Design review of the part built by this model. Coordinates are the model's own, in mm. Face numbers are marked on the shaded views. A direction names the side the tool comes from. Round coordinates to 2 decimals unless told otherwise and drop trailing zeros. Order: outer loops, then holes, each group sorted by start corner. A loop starts at its lowest first (then second) coordinate and runs counter-clockwise, first axis right, second up. Notation, with made-up numbers: M 64,5 L 75,5 A19 cw 75,26 Z; hole C -6.5,-40 d10. An arc over 180 degrees is marked long. Use a Markdown table: item, result. Add a question column.
(1) The part is to be moulded in two halves that separate along Y. For the marked faces 1, 2, 3 and 4, say which applies: released by +Y, released by -Y, zero draft, split by the parting line, or undercut.
(2) Take a section at C-C (z = 6.5). Write out the cut boundary in (x, y).
(3) Take a section at A-A (y = -29). Write out the cut boundary in (x, z), then the cut area to 3 significant figures.
(4) Machinability: for the marked faces 5, 6 and 7, which of the approach directions +Z, -Z, +X, -X, +Y, -Y give a long, thin tool a straight path to every point of the face, cutting with its end or side? Answer none if there is none.
(5) For pin 1 (4 mm diameter, centred on x = 37.5, z = 5.5, fed in from -Y); pin 2 (2.5 mm diameter, centred on x = -41, z = 6, fed in from -Y); pin 3 (1 mm diameter, centred on y = -3, z = 5.5, fed in from -X); pin 4 (4 mm diameter, centred on x = -30, y = -29.5, fed in from +Z), all flat-tipped, find the tip position at first contact; note any pin that passes through.
(6) Take a section at D-D (x = -36). Write out the cut boundary in (y, z), then the cut area to 3 significant figures.
(7) Take a section at B-B (y = -16). Write out the cut boundary in (x, z).
(8) To check wall thickness, follow probe 1 along X at (y, z) = (-28, 6); probe 2 along Y at (x, z) = (0.5, 6); probe 3 along X at (y, z) = (-10, 1.75). State the ranges of each line that lie inside material, in increasing order. Write a range as from..to.
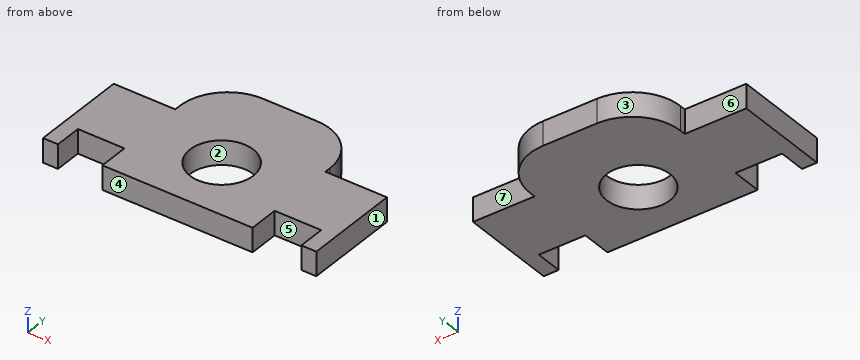
```python
from build123d import *

# Parameters (mm, degrees)
SKETCH2_W           = 70
SKETCH2_H           = 51
SKETCH2_R           = 10.55
BOSS_EXTRUDE1_DEPTH = 8
SKETCH3_W           = 10
SKETCH3_H           = 10
CUT_EXTRUDE1_DEPTH  = 53.436444721
SKETCH5_W           = 5.5
SKETCH5_H           = 8
BOSS_EXTRUDE2_DEPTH = 23
SKETCH5_3_W         = 5
SKETCH5_3_H         = 8
BOSS_EXTRUDE3_DEPTH = 32
SKETCH5_5_W         = 5
SKETCH5_5_H         = 8
BOSS_EXTRUDE4_DEPTH = 32
SKETCH5_6_W         = 5.5
SKETCH5_6_H         = 8
BOSS_EXTRUDE5_DEPTH = 23


with BuildPart() as part:
    # Sketch2 → Boss-Extrude1 (new body)
    with BuildSketch(Plane.XY):
        with Locations((1.074313409, -11.705169628)):
            Rectangle(SKETCH2_W, SKETCH2_H)
        with Locations((1.074313409, -17.205169628)):
            Circle(SKETCH2_R, mode=Mode.SUBTRACT)
    extrude(amount=BOSS_EXTRUDE1_DEPTH)

    # Sketch3 → Cut-Extrude1 (cut, through all)
    with BuildSketch(Plane.XY.offset(8)):
        with Locations((31.074313409, -32.205169628)):
            Rectangle(SKETCH3_W, SKETCH3_H)
        with Locations((-28.925686591, -32.205169628)):
            Rectangle(SKETCH3_W, SKETCH3_H)
        with BuildLine():
            Line((26.074313409, -4.205169628), (36.074313409, -4.205169628))
            Line((36.074313409, -4.205169628), (36.074313409, 13.794830372))
            Line((36.074313409, 13.794830372), (10.074313409, 13.794830372))
            ThreePointArc((10.074313409, 13.794830372), (21.388021908, 9.108538871), (26.074313409, -2.205169628))
            Line((26.074313409, -2.205169628), (26.074313409, -4.205169628))
        make_face()
        with BuildLine():
            Line((-33.925686591, 13.794830372), (-33.925686591, -4.205169628))
            Line((-33.925686591, -4.205169628), (-23.925686591, -4.205169628))
            Line((-23.925686591, -4.205169628), (-23.925686591, -2.205169628))
            ThreePointArc((-23.925686591, -2.205169628), (-19.23939509, 9.108538871), (-7.925686591, 13.794830372))
            Line((-7.925686591, 13.794830372), (-33.925686591, 13.794830372))
        make_face()
    extrude(amount=-CUT_EXTRUDE1_DEPTH, mode=Mode.SUBTRACT)

    # Sketch5 → Boss-Extrude2 (add)
    with BuildSketch(Plane(origin=(0, -4.205169628, 0), x_dir=(1, 0, 0), z_dir=(0, 1, 0))):
        with Locations((-36.675686591, -4)):
            Rectangle(SKETCH5_W, SKETCH5_H)
    extrude(amount=-BOSS_EXTRUDE2_DEPTH)

    # Sketch5_3 → Boss-Extrude3 (add)
    with BuildSketch(Plane(origin=(0, -4.205169628, 0), x_dir=(1, 0, 0), z_dir=(0, 1, 0))):
        with Locations((-41.925686591, -4)):
            Rectangle(SKETCH5_3_W, SKETCH5_3_H)
    extrude(amount=-BOSS_EXTRUDE3_DEPTH)



with BuildPart() as body_2:
    # Sketch5_5 → Boss-Extrude4 (new body)
    with BuildSketch(Plane(origin=(0, -4.205169628, 0), x_dir=(1, 0, 0), z_dir=(0, 1, 0))):
        with Locations((44.074313409, -4)):
            Rectangle(SKETCH5_5_W, SKETCH5_5_H)
    extrude(amount=-BOSS_EXTRUDE4_DEPTH)


with BuildPart() as part_1:
    add(part.part)

    add(body_2.part)  # Boss-Extrude5 merges body 2
    # Sketch5_6 → Boss-Extrude5 (add)
    with BuildSketch(Plane(origin=(0, -4.205169628, 0), x_dir=(1, 0, 0), z_dir=(0, 1, 0))):
        with Locations((38.824313409, -4)):
            Rectangle(SKETCH5_6_W, SKETCH5_6_H)
    extrude(amount=-BOSS_EXTRUDE5_DEPTH)


solid = part_1.part
```
Verdict:
| question | item | result |
|---|---|---|
| 1 | face 1 | zero draft |
| 1 | face 2 | undercut |
| 1 | face 3 | released by +Y |
| 1 | face 4 | released by -Y |
| 2 | outline | M -44.43,-36.21 L -39.43,-36.21 L -39.43,-27.21 L -23.93,-27.21 L -23.93,-37.21 L 26.07,-37.21 L 26.07,-27.21 L 41.57,-27.21 L 41.57,-36.21 L 46.57,-36.21 L 46.57,-4.21 L 26.07,-4.21 L 26.07,-2.21 A16 ccw 10.07,13.79 L -7.93,13.79 A16 ccw -23.93,-2.21 L -23.93,-4.21 L -44.43,-4.21 Z; hole C 1.07,-17.21 d21.1 |
| 3 | outline | M -44.43,0 L -39.43,0 L -39.43,8 L -44.43,8 Z; M -23.93,0 L 26.07,0 L 26.07,8 L -23.93,8 Z; M 41.57,0 L 46.57,0 L 46.57,8 L 41.57,8 Z |
| 3 | area | 480 mm^2 |
| 4 | face 5 | +Z, -Z, -Y |
| 4 | face 6 | +Z, -Z, -X, +Y |
| 4 | face 7 | +Z, -Z, +X, +Y |
| 5 | pin 1 | stops at y = -27.21 |
| 5 | pin 2 | stops at y = -36.21 |
| 5 | pin 3 | stops at x = -23.93 |
| 5 | pin 4 | passes through |
| 6 | outline | M -27.21,0 L -4.21,0 L -4.21,8 L -27.21,8 Z |
| 6 | area | 184 mm^2 |
| 7 | outline | M -44.43,0 L -9.41,0 L -9.41,8 L -44.43,8 Z; M 11.56,0 L 46.57,0 L 46.57,8 L 11.56,8 Z |
| 8 | probe 1 | x = -44.43..-39.43, -23.93..26.07, 41.57..46.57 |
| 8 | probe 2 | y = -37.21..-27.74, -6.67..13.79 |
| 8 | probe 3 | x = -44.43..-6.63, 8.78..46.57 |
